Autodesk Fusion 360 part; units mm, degrees
sketch "Sketch1" plane through (0, 0, 0) normal (0, 1, 0) x (1, 0, 0)
  line L0 (0, 12.575) -> (27.15, 12.575) construction
  line L1 (27.15, 12.575) -> (27.15, -8.575)
  line L2 (23.15, -12.575) -> (0, -12.575)
  line L3 (27.15, 12.575) -> (33.15, 12.575)
  line L4 (33.15, 12.575) -> (33.15, 6.575)
  line L5 (33.15, 6.575) -> (27.15, 6.575)
  line L6 (27.15, 6.575) -> (27.15, 12.575)
  line L7 (0, -12.575) -> (0, 12.575) construction
  circle A0 centre (30.15, 9.575) radius 1.425
  line L8 (27.15, 6.575) -> (33.15, 12.575) construction
  arc A1 (23.15, -12.575) -> (27.15, -8.575) centre (23.15, -8.575) ccw
  line L9 (-27.15, 12.575) -> (-27.15, -8.575)
  line L10 (-33.15, 6.575) -> (-27.15, 6.575)
  circle A2 centre (-30.15, 9.575) radius 1.425
  line L11 (-27.15, 12.575) -> (-33.15, 12.575)
  line L12 (-33.15, 12.575) -> (-33.15, 6.575)
  line L13 (-23.15, -12.575) -> (0, -12.575)
  arc A3 (-27.15, -8.575) -> (-23.15, -12.575) centre (-23.15, -8.575) ccw
  line L14 (-27.15, 0) -> (27.15, 0) construction
  line L15 (-27.15, 12.575) -> (-27.15, 22.575)
  line L16 (-27.15, 22.575) -> (27.15, 22.575)
  line L17 (27.15, 22.575) -> (27.15, 12.575)
  line L18 (22, 18.575) -> (20, 18.575)
  line L19 (22, -8.575) -> (22, 18.575)
  line L20 (20, -8.575) -> (22, -8.575)
  line L21 (20, 18.575) -> (20, -8.575)
  line L22 (16, -8.575) -> (16, 18.575)
  line L23 (14, 18.575) -> (14, -8.575)
  line L24 (14, -8.575) -> (16, -8.575)
  line L25 (16, 18.575) -> (14, 18.575)
  line L26 (-4, 17.575) -> (4, 17.575)
  line L27 (-4, 17.575) -> (-9, 22.575)
  line L28 (4, 17.575) -> (9, 22.575)
  line L29 (11, 13.4) -> (11, -3.4)
  line L30 (-11, -3.4) -> (-11, 13.4)
  line L31 (-11, 11.4) -> (11, 11.4)
  line L32 (-11, -1.4) -> (11, -1.4)
  line L33 (-11, 13.4) -> (11, 13.4)
  line L34 (-11, -3.4) -> (11, -3.4)
  line L35 (-11, 5) -> (11, 5) construction
  line L36 (-14, -8.575) -> (-16, -8.575)
  line L37 (-14, 18.575) -> (-14, -8.575)
  line L38 (-16, -8.575) -> (-16, 18.575)
  line L39 (-16, 18.575) -> (-14, 18.575)
  line L40 (-22, 18.575) -> (-20, 18.575)
  line L41 (-20, 18.575) -> (-20, -8.575)
  line L42 (-22, -8.575) -> (-22, 18.575)
  line L43 (-20, -8.575) -> (-22, -8.575)
  circle A4 centre (3.52, 8.86) radius 0.925
  circle A5 centre (8.6, 1.14) radius 0.925
  circle A6 centre (-8.6, 8.86) radius 0.925
  circle A7 centre (-3.52, 1.14) radius 0.925
  point P0 (0, 17.575)
  point P1 (0, 5)
  dimension "d1" = 6
  dimension "d2" = 6
  dimension "d4" = 33.15
  dimension "d5" = 2.85
  dimension "d6" = 4
  dimension "d16" = 10
  dimension "d18" = 25.15
  dimension "d25" = 5
  dimension "d26" = 45
  dimension "d27" = 45
  dimension "d28" = 8
  dimension "d29" = 22
  dimension "d32" = 12.8
  dimension "d33" = 2
  dimension "d34" = 2
  dimension "d36" = 5
  dimension "d37" = 2
  dimension "d38" = 27.15
  dimension "d39" = 14
  dimension "d40" = 4
  dimension "d41" = 4
  dimension "d56" = 2.4
  dimension "d57" = 2.54
  dimension "d58" = 2.54
  dimension "d59" = 7.48
  dimension "d60" = 1.85
  dimension "d61" = 2.4
  dimension "d62" = 2.54
  dimension "d63" = 7.48
  dimension "d64" = 2.54
extrude "Extrude1" add sketch "Sketch1" along normal blind 2 contours L1 L3 L4 L5 L6 | L1 L2 L6 A1 L9 L13 A3 L15 L16 L17 L26 L27 L28 | L9 L10 L11 L12 | L29 L30 L31 L33 | L29 L30 L31 L32 | L29 L30 L32 L34 | A4 | A5 | A6 | A7
extrude "Extrude2" add sketch "Sketch1" along normal blind 10 from surface at 2 contours L29 L30 L31 L33 | L29 L30 L31 L32 | L29 L30 L32 L34 | A4 | A5 | A6 | A7
extrude "Extrude3" cut sketch "Sketch1" against normal blind 2.5 from surface at 12 contours L29 L30 L31 L32 | A4 | A5 | A6 | A7
extrude "Extrude4" cut sketch "Sketch1" against normal blind 8 from surface at 9.5 contours A4 | A5 | A6 | A7
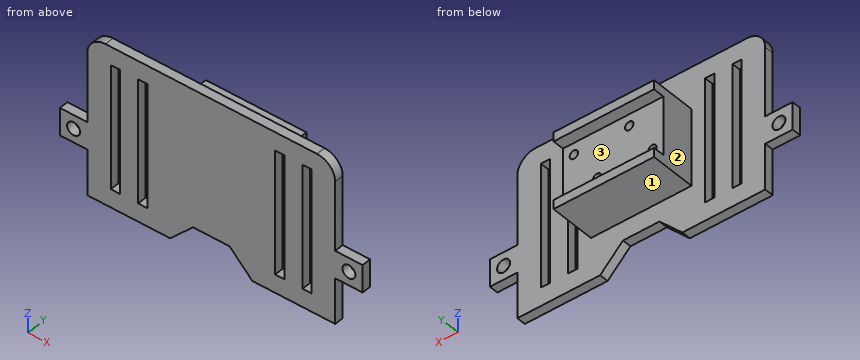
CAD build for the part. Positions are in the model's coordinates, mm. Face numbers are marked on the shaded views. A direction names the side the tool comes from. Round coordinates to 2 decimals unless told otherwise and drop trailing zeros. Loops run counter-clockwise (first coordinate to the right, second up) from the corner with the lowest first, then second, coordinate; pieces in that order, holes last. Notation, with made-up numbers: M 12.5,25.25 L 18.5,25.25 A11 cw 18.5,44.25 Z; hole C -7.75,88.5 d4. An arc over 180 degrees is marked long. Use a Markdown table: item, result. Add a question column.
(1) Cut at A-A (x = -30.15). Give the cut face in (y, z) (3 decimals).
(2) Flat gauge pins, fed straight in: pin 1 (2 mm diameter, centred on y = 1, z = 1.5, fed in from -X); pin 2 (5 mm diameter, centred on x = 0.5, y = 9.5, fed in from -Z); pin 3 (1.5 mm diameter, centred on x = -19, y = 3.5, fed in from +Z); pin 4 (4 mm diameter, centred on x = -21.5, z = 4.5, fed in from +Y). Where does each tip first touch, or does it go through?
(3) Cut at D-D (y = 10.75). Give the cut face in (x, z), and give its area (3 significant figures).
(4) Which spindle directions (+Z, -Z, +X, -X, +Y, -Y) get a long thin tool onto all of the face, cutting with end or side? Do the marked faces 1, 2 and 3. Say none if no direction does.
(5) Cut at B-B (z = 6.5). Give the cut face in (x, y).
(6) Drill centre lines: line 1 (X direction, y = 4.75, z = -1.14) (3 decimals); line 2 (Z direction, x = -30.15, y = 1) (3 decimals); line 3 (Z direction, x = -3.52, y = 5) (3 decimals). Where is each one in solid material? Low to high.
(7) Cut at C-C (y = 4.75). Give the cut face in (x, z) (3 decimals), and give its area (3 significant figures).
Geometry says:
| question | item | result |
|---|---|---|
| 1 | outline | M 0,-12.575 L 2,-12.575 L 2,-11 L 0,-11 Z; M 0,-8.15 L 2,-8.15 L 2,-6.575 L 0,-6.575 Z |
| 2 | pin 1 | stops at x = -27.15 |
| 2 | pin 2 | stops at z = -13.4 |
| 2 | pin 3 | passes through |
| 2 | pin 4 | stops at y = 2 |
| 3 | outline | M -11,-13.4 L 11,-13.4 L 11,-11.4 L -11,-11.4 Z; M -11,1.4 L 11,1.4 L 11,3.4 L -11,3.4 Z |
| 3 | area | 88.0 mm² |
| 4 | face 1 | -Z, +X, -X, +Y |
| 4 | face 2 | +Z, -Z, -X, +Y |
| 4 | face 3 | +X, -X, +Y |
| 5 | outline | M -27.15,0 L -22,0 L -22,2 L -27.15,2 Z; M -20,0 L -16,0 L -16,2 L -20,2 Z; M -14,0 L 14,0 L 14,2 L -14,2 Z; M 16,0 L 20,0 L 20,2 L 16,2 Z; M 22,0 L 27.15,0 L 27.15,2 L 22,2 Z |
| 6 | line 1 | x = -11 to -4.445, -2.595 to 7.675, 9.525 to 11 |
| 6 | line 2 | z = -12.575 to -11, -8.15 to -6.575 |
| 6 | line 3 | z = -13.4 to -2.065, -0.215 to 3.4 |
| 7 | outline | M -11,-13.4 L 11,-13.4 L 11,3.4 L -11,3.4 Z; hole C -8.6,-8.86 d1.85; hole C -3.52,-1.14 d1.85; hole C 3.52,-8.86 d1.85; hole C 8.6,-1.14 d1.85 |
| 7 | area | 359 mm² |
